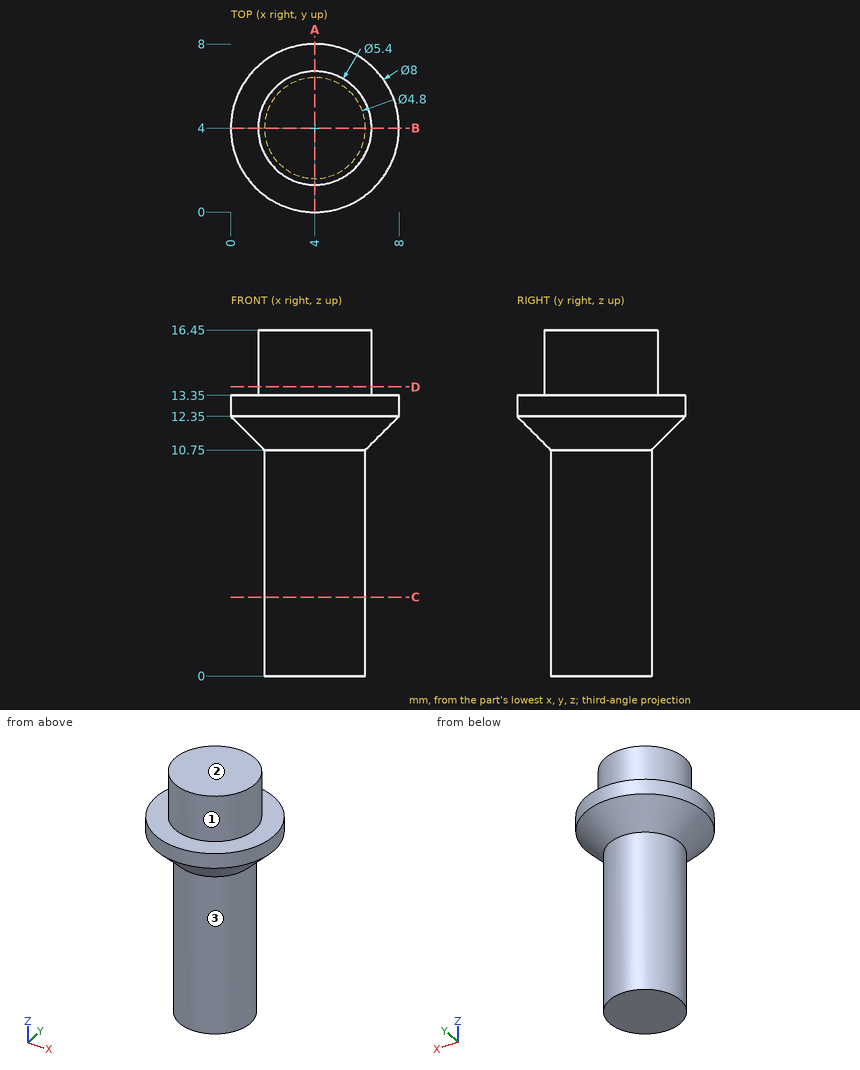
Verification items for this drawing (mm, ordinates from the low corner). A direction names the side the tool comes from. Round coordinates to 2 decimals unless told otherwise and drop trailing zeros. Loops run counter-clockwise (first coordinate to the right, second up) from the corner with the lowest first, then second, coordinate; pieces in that order, holes last. Notation, with made-up numbers: (-3, 47) -> (21, 47) arc R3 cw to (21, 51) -> close; hole circle Ø1 at (15.5, 66). An arc over 180 degrees is marked (long way). Write item = value, one per line. Start each with the question number.
1) Sectioned sample at A-A, the plane x = 4. Record the cut outline in (y, z), plus the area to 3 significant figures.
2) Gauge pin test, flat end, axial feed: pin 1 Ø3 at (x, y) = (6.5, 3) entering from -Z. Record the tip position at first contact, or that the pin passes through.
3) Set-up check for the marked faces 1, 2 and 3: record each of +Z, -Z, +X, -X, +Y, -Y from which the full face is reachable in a straight line by a thin tool's end or side.
4) Sectioned sample at D-D, the plane z = 13.75. Record the cut outline in (x, y), plus the area to 3 significant figures.
5) Thickness scan on probe 1 along X at (y, z) = (4.5, 13.5); probe 2 along Y at (x, z) = (6, 1); probe 3 along Y at (x, z) = (5, 9.25). Record the ranges inside material, lowest first.
6) Sectioned sample at C-C, the plane z = 3.75. Record the cut outline in (x, y), plus the area to 3 significant figures.
Results are:
q1.outline = (0, 12.35) -> (1.6, 10.75) -> (1.6, 0) -> (6.4, 0) -> (6.4, 10.75) -> (8, 12.35) -> (8, 13.35) -> (6.7, 13.35) -> (6.7, 16.45) -> (1.3, 16.45) -> (1.3, 13.35) -> (0, 13.35) -> close
q1.area = 86.6 mm^2
q2.pin_1 = 0
q3.face_1 = +Z
q3.face_2 = +Z, +X, -X, +Y, -Y
q3.face_3 = -Z
q4.outline = circle Ø5.4 at (4, 4)
q4.area = 22.9 mm^2
q5.probe_1 = 1.35 to 6.65
q5.probe_2 = 2.67 to 5.33
q5.probe_3 = 1.82 to 6.18
q6.outline = circle Ø4.8 at (4, 4)
q6.area = 18.1 mm^2
